Source: CAD feature listing. Evaluate the final solid. Frame: model axes, mm. Coordinates: 2 decimals unless noted, no trailing zeros. Order: outer loops, then holes, each group sorted by start corner. A loop starts at its lowest first (then second) coordinate and runs counter-clockwise, first axis right, second up.
Item 1: Section B-B on y = 8. Return the cut outline in (x, z), then the cut area to 3 significant figures.
Item 2: Contact query for flat-ended pins moving along their axis: P1, Ø0.9, axis at y = -4, z = 1.5, coming from the +X side; P2, Ø1.5, axis at x = 41.5, z = 2, coming from the -Y side; P3, Ø0.9, axis at x = 45, z = 1, coming from the +Y side. Output: stop coordinate, or through.
Item 3: Section C-C on z = 1.8. Return the cut outline in (x, y).
Item 4: Ray query, line 1 (X direction, y = 10.5, z = 0.1); line 2 (Y direction, x = 25, z = 1.3); line 3 (Y direction, x = 35.5, z = 0.4). Return the intervals inside material, ascending.
Item 5: Section A-A on x = 35. Return the cut outline in (y, z).
from build123d import *

# Parameters (mm, degrees)
BOSS_EXTRUDE1_DEPTH = 3
SKETCH2_W           = 15
SKETCH2_H           = 12
CUT_EXTRUDE1_DEPTH  = 68.245817714
FILLET1_R           = 1


with BuildPart() as part:
    # Sketch1 → Boss-Extrude1 (new body)
    with BuildSketch(Plane.XY):
        Polygon((0, 0), (0, 45), (12, 45), (12, 48), (32, 48), (32, 45), (47, 45), (47, 27.5), (44, 27.5), (44, 17.5), (47, 17.5), (47, 0), (32, 0), (32, -6), (12, -6), (12, 0), align=None)
    extrude(amount=BOSS_EXTRUDE1_DEPTH)

    # Sketch2 → Cut-Extrude1 (cut, through all)
    with BuildSketch(Plane.XY.offset(3)):
        with Locations((31.5, 11)):
            Rectangle(SKETCH2_W, SKETCH2_H)
    extrude(amount=-CUT_EXTRUDE1_DEPTH, mode=Mode.SUBTRACT)

    # Fillet1
    fillet1_edges = [part.edges().sort_by_distance(p)[0] for p in [
        (24, 5, 1.5),
        (24, 17, 1.5),
        (39, 17, 1.5),
        (39, 5, 1.5),
    ]]
    fillet(fillet1_edges, radius=FILLET1_R)


solid = part.part
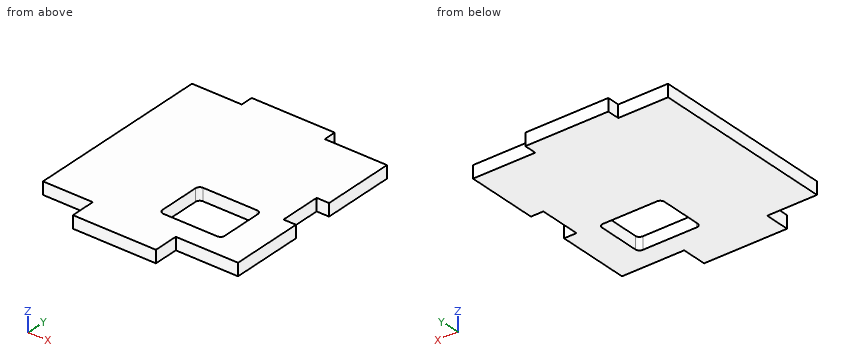
Answer list:
1. outline: (0, 0) - (24, 0) - (24, 3) - (0, 3) - close; (39, 0) - (47, 0) - (47, 3) - (39, 3) - close
1. area: 96.0 mm2
2. P1: stops at x = 32
2. P2: stops at y = 0
2. P3: stops at y = 45
3. outline: (0, 0) - (12, 0) - (12, -6) - (32, -6) - (32, 0) - (47, 0) - (47, 17.5) - (44, 17.5) - (44, 27.5) - (47, 27.5) - (47, 45) - (32, 45) - (32, 48) - (12, 48) - (12, 45) - (0, 45) - close; hole (24, 6) arc R1 ccw to (25, 5) - (38, 5) arc R1 ccw to (39, 6) - (39, 16) arc R1 ccw to (38, 17) - (25, 17) arc R1 ccw to (24, 16) - close
4. line 1: x = 0 to 24, 39 to 47
4. line 2: y = -6 to 5, 17 to 48
4. line 3: y = 0 to 5, 17 to 45
5. outline: (0, 0) - (5, 0) - (5, 3) - (0, 3) - close; (17, 0) - (45, 0) - (45, 3) - (17, 3) - close
